```python
from build123d import *

# Parameters (mm, degrees)
BOSS_EXTRUDE1_OUTLINE_W   = 25.6
BOSS_EXTRUDE1_OUTLINE_H   = 50.75
BOSS_EXTRUDE1_OUTLINE_R   = 2.15
BOSS_EXTRUDE1_OUTLINE_R_2 = 2.1
BOSS_EXTRUDE1_DEPTH       = 4.45
FILLET1_R                 = 2


# Read off the part's stored shape, not the designer's step: Boss-Extrude1
with BuildPart() as part:
    # Boss-Extrude1 outline → Boss-Extrude1 (new body)
    with BuildSketch(Plane.XY):
        Polygon((-4.45, 6.2), (-4.45, -8.375), (-10.9, -8.375), (-10.9, -68.025), (23.6, -68.025), (23.6, -8.375), (17.15, -8.375), (17.15, 6.2), align=None)
        with Locations((6.35, -38.2)):
            Rectangle(BOSS_EXTRUDE1_OUTLINE_W, BOSS_EXTRUDE1_OUTLINE_H, mode=Mode.SUBTRACT)
        Circle(BOSS_EXTRUDE1_OUTLINE_R, mode=Mode.SUBTRACT)
        with Locations((12.7, 0)):
            Circle(BOSS_EXTRUDE1_OUTLINE_R_2, mode=Mode.SUBTRACT)
    extrude(amount=BOSS_EXTRUDE1_DEPTH)

    # Fillet1
    fillet1_edges = [part.edges().sort_by_distance(p)[0] for p in [
        (-10.9, -8.375, 2.225),
        (-10.9, -68.025, 2.225),
        (23.6, -68.025, 2.225),
        (23.6, -8.375, 2.225),
        (17.15, -8.375, 2.225),
        (17.15, 6.2, 2.225),
        (-4.45, 6.2, 2.225),
        (-4.45, -8.375, 2.225),
    ]]
    fillet(fillet1_edges, radius=FILLET1_R)


solid = part.part
```
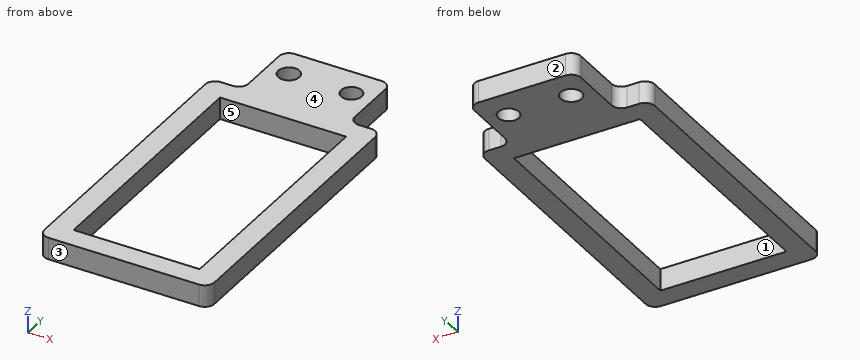
For this review, take the finished solid that the model builds, in its own axes (mm). Face numbers are marked on the shaded views. A direction names the side the tool comes from. Round coordinates to 2 decimals unless told otherwise and drop trailing zeros. Write each loop counter-clockwise with the first axis right and the second up, starting at its lowest first coordinate (ties: lowest second). Pieces come first, ordered by that corner, then holes. Notation, with made-up numbers: (44, -4.75) -> (59, -4.75) arc R27 ccw to (59, 20.25) -> close; hole circle Ø10 at (89, 33.25). An arc over 180 degrees is marked (long way). One line per question, with ' | ' between items. Start each with the question number.
1) Mouldability with a two-part tool opening along Y and no side actions: class the marked faces 1, 2 and 3 as +Y half, -Y half, draft (parallel to the pull), parting line (faces both ways), or undercut.
2) Machinability: for the marked faces 4 and 5, which of the approach directions +Z, -Z, +X, -X, +Y, -Y give a long, thin tool a straight path to every point of the face, cutting with its end or side? Answer none if there is none.
3) Wall thickness on line 1 along Y through (x, z) = (0, 1.3) (3 decimals); line 2 along X through (y, z) = (1.5, 1.65); line 3 along Y through (x, z) = (3.5, 1.8) (3 decimals): over which ranges is each line inside the solid? List them lowest first.
4) For pin 1 Ø5 at (x, y) = (12.7, 0) entering from -Z; pin 2 Ø1 at (x, z) = (16.5, 2.5) entering from +Y; pin 3 Ø0.7 at (x, z) = (20, 2) entering from +Y (3 decimals); pin 4 Ø2 at (y, z) = (0, 1.5) entering from -X, all flat-tipped, find the tip position at first contact; note any pin that passes through.
5) Add section A-A (x = 12.7). Write out the cut boundary in (y, z) (3 decimals).
6) Add section C-C (x = 4). Write out the cut boundary in (y, z) (3 decimals), and give its area (3 significant figures).
7) Add section B-B (y = -16). Write out the cut boundary in (x, z).
8) Add section D-D (y = 0). Write out the cut boundary in (x, z).
Reported:
1) face 1: undercut | face 2: +Y half | face 3: -Y half
2) face 4: +Z, +X, -X, +Y, -Y | face 5: +Z, -Z
3) line 1: y = -68.025 to -63.575, -12.825 to -2.15, 2.15 to 6.2 | line 2: x = -4.45 to -1.54, 1.54 to 11.23, 14.17 to 17.15 | line 3: y = -68.025 to -63.575, -12.825 to 6.2
4) pin 1: stops at z = 0 | pin 2: stops at y = 6.01 | pin 3: stops at y = -8.375 | pin 4: stops at x = -4.45
5) outline: (-68.025, 0) -> (-63.575, 0) -> (-63.575, 4.45) -> (-68.025, 4.45) -> close; (-12.825, 0) -> (-2.1, 0) -> (-2.1, 4.45) -> (-12.825, 4.45) -> close; (2.1, 0) -> (6.2, 0) -> (6.2, 4.45) -> (2.1, 4.45) -> close
6) outline: (-68.025, 0) -> (-63.575, 0) -> (-63.575, 4.45) -> (-68.025, 4.45) -> close; (-12.825, 0) -> (6.2, 0) -> (6.2, 4.45) -> (-12.825, 4.45) -> close | area: 104 mm²
7) outline: (-10.9, 0) -> (-6.45, 0) -> (-6.45, 4.45) -> (-10.9, 4.45) -> close; (19.15, 0) -> (23.6, 0) -> (23.6, 4.45) -> (19.15, 4.45) -> close
8) outline: (-4.45, 0) -> (-2.15, 0) -> (-2.15, 4.45) -> (-4.45, 4.45) -> close; (2.15, 0) -> (10.6, 0) -> (10.6, 4.45) -> (2.15, 4.45) -> close; (14.8, 0) -> (17.15, 0) -> (17.15, 4.45) -> (14.8, 4.45) -> close
